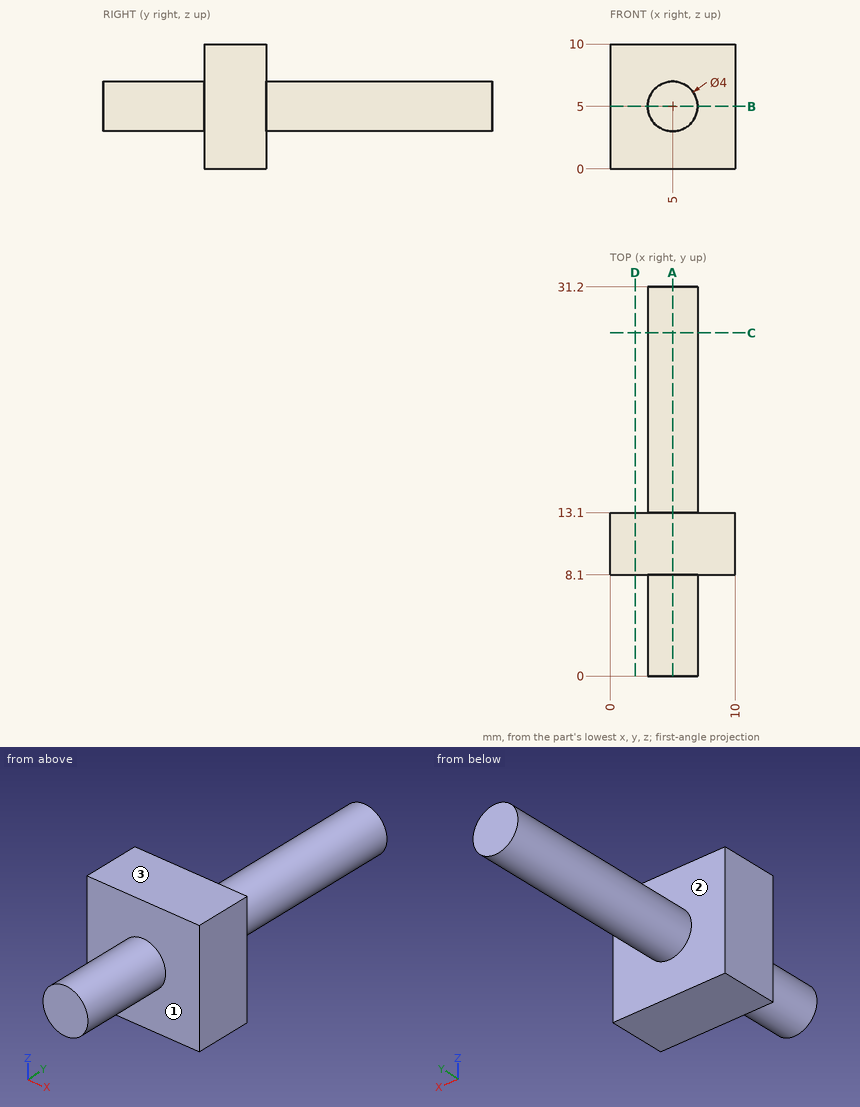
Check sheet for the drawn part. Datum: minimum x, y, z corner. Units: mm. A direction names the side the tool comes from. Give positions to 0.01 mm unless a question says otherwise; leave off trailing zeros. Write each loop counter-clockwise with the first axis right and the second up, starting at its lowest first coordinate (ties: lowest second). Pieces come first, ordered by that corner, then holes. Notation, with made-up numbers: (-18.5, 54.5) -> (19.5, 54.5) arc R26 ccw to (19.5, 87.5) -> close; hole circle Ø11 at (66, 42.5). An arc over 180 degrees is marked (long way). Use one line per item in the form item = value. Start each with the question number.
1. Section check C-C (y = 27.5). Record the cut outline in (x, z).
2. Go/stop test with flat-tipped pins: P1, Ø4, axis at x = 4.5, z = 8.5, coming from the -Y side; P2, Ø1.5, axis at x = 5, y = 3.5, coming from the -Z side; P3, Ø2, axis at x = 3.5, y = 23.5, coming from the -Z side; P4, Ø6, axis at x = 5.5, y = 17.5, coming from the +Z side. Record where each tip stops, or that it passes through.
3. Section check B-B (z = 5). Record the cut outline in (x, y).
4. Section check D-D (x = 2). Record the cut outline in (y, z), and give its area (3 significant figures).
5. Thickness scan on line 1 along Y through (x, z) = (2.75, 7); line 2 along X through (y, z) = (14.5, 4.75); line 3 along Z through (x, y) = (6.5, 21.5). Record the ranges inside material, lowest first. Write a range as from..to.
6. Section check A-A (x = 5). Record the cut outline in (y, z), and give its area (3 significant figures).
7. Access from +Z, -Z, +X, -X, +Y, -Y to the whole of each face (thin tool, end or side, straight path). Record for the marked faces 1, 2 and 3.
Conclusion:
q1.outline = circle Ø4 at (5, 5)
q2.P1 = 0
q2.P2 = 3
q2.P3 = 3.06
q2.P4 = 7
q3.outline = (0, 8.1) -> (3, 8.1) -> (3, 0) -> (7, 0) -> (7, 8.1) -> (10, 8.1) -> (10, 13.1) -> (7, 13.1) -> (7, 31.2) -> (3, 31.2) -> (3, 13.1) -> (0, 13.1) -> close
q4.outline = (8.1, 0) -> (13.1, 0) -> (13.1, 10) -> (8.1, 10) -> close
q4.area = 50.0 mm²
q5.line_1 = 8.1..13.1
q5.line_2 = 3.02..6.98
q5.line_3 = 3.68..6.32
q6.outline = (0, 3) -> (8.1, 3) -> (8.1, 0) -> (13.1, 0) -> (13.1, 3) -> (31.2, 3) -> (31.2, 7) -> (13.1, 7) -> (13.1, 10) -> (8.1, 10) -> (8.1, 7) -> (0, 7) -> close
q6.area = 155 mm²
q7.face_1 = -Y
q7.face_2 = +Y
q7.face_3 = +Z, +X, -X, +Y, -Y
